Check sheet for the drawn part. Datum: minimum x, y, z corner. Units: mm. A direction names the side the tool comes from. Coordinates: 2 decimals unless noted, no trailing zeros. Order: outer loops, then holes, each group sorted by start corner. A loop starts at its lowest first (then second) coordinate and runs counter-clockwise, first axis right, second up.
Q1. Depth check by flat-ended pin: P1, Ø3, axis at x = 4.5, y = 18, coming from the +Z side; P2, Ø6, axis at x = 21, z = 9, coming from the +Y side; P3, Ø15.5, axis at x = 9, y = 10.5, coming from the +Z side; P4, Ø0.5, axis at x = 28, z = 5.5, coming from the +Y side. Enter the tip coordinate at first touch or a pass-through.
Q2. Cross-section at A-A, the plane y = 28.6. Record the boundary of the cut face in (x, z).
Q3. Cross-section at B-B, the plane x = 29.9. Record the boundary of the cut face in (y, z).
Q4. Thickness scan on line 1 (Y direction, x = 29.9, z = 4.2); line 2 (Y direction, x = 10.5, z = 2.75); line 3 (Z direction, x = 16, y = 17.5). Record the ranges inside material, lowest first.
Q5. Cross-section at C-C, the plane x = 24.5. Record the boundary of the cut face in (y, z), and give its area (3 significant figures).
Q6. Set-up check for the marked faces 1, 2, 3, 4 and 5: record each of +Z, -Z, +X, -X, +Y, -Y from which the full face is reachable in a straight line by a thin tool's end or side.
Q7. Cross-section at D-D, the plane z = 8.5. Record the boundary of the cut face in (x, y).
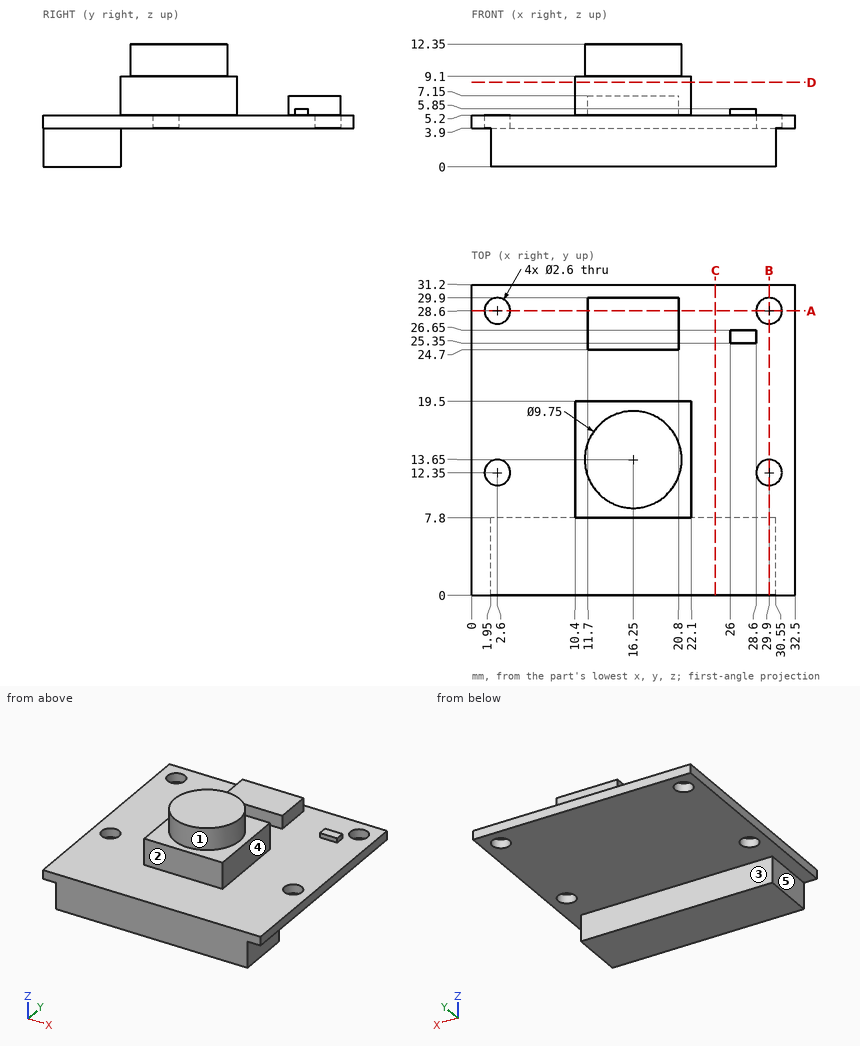
Check values:
1. P1: stops at z = 5.2
1. P2: stops at y = 29.9
1. P3: stops at z = 12.35
1. P4: stops at y = 26.65
2. outline: (0, 3.9) - (1.3, 3.9) - (1.3, 5.2) - (0, 5.2) - close; (3.9, 3.9) - (28.6, 3.9) - (28.6, 5.2) - (20.8, 5.2) - (20.8, 7.15) - (11.7, 7.15) - (11.7, 5.2) - (3.9, 5.2) - close; (31.2, 3.9) - (32.5, 3.9) - (32.5, 5.2) - (31.2, 5.2) - close
3. outline: (0, 0) - (7.8, 0) - (7.8, 3.9) - (11.05, 3.9) - (11.05, 5.2) - (0, 5.2) - close; (13.65, 3.9) - (27.3, 3.9) - (27.3, 5.2) - (13.65, 5.2) - close; (29.9, 3.9) - (31.2, 3.9) - (31.2, 5.2) - (29.9, 5.2) - close
4. line 1: y = 0 to 11.05, 13.65 to 27.3, 29.9 to 31.2
4. line 2: y = 0 to 7.8
4. line 3: z = 3.9 to 12.35
5. outline: (0, 0) - (7.8, 0) - (7.8, 3.9) - (31.2, 3.9) - (31.2, 5.2) - (0, 5.2) - close
5. area: 71.0 mm2
6. face 1: +Z
6. face 2: +Z, +X, -X, -Y
6. face 3: -Z, +X, -X, +Y
6. face 4: +Z, +X, +Y, -Y
6. face 5: -Z, -X, +Y, -Y
7. outline: (10.4, 7.8) - (22.1, 7.8) - (22.1, 19.5) - (10.4, 19.5) - close
